Could you check a few things on this model? Use its own coordinates, in mm. A direction names the side the tool comes from. Give positions to 0.01 mm unless a question says otherwise; leave off trailing zeros. Loops run counter-clockwise (first coordinate to the right, second up) from the corner with the lowest first, then second, coordinate; pieces in that order, holes last. Notation, with made-up numbers: M 22.25,12.5 L 42.25,12.5 A17 cw 42.25,32.5 Z; hole C 29.5,73 d8. An arc over 180 degrees is marked long. Return JSON: item names as keys, results as strings. Group by question number.
1. If we mould it in two halves opening along X, with no side actions, what happens to faces 4 (the flat face through (39, 3, 10)), 5 (the flat face through (-76.2, -3, 5)), 6 (the flat face through (-2, 3, 10)), 7 (the flat face through (49, 3, 15))? For each: +X half, -X half, draft (parallel to the pull), parting line (faces both ways), or undercut.
2. If we section it at B-B (x = 0): Write out the boundary of the cut face in (y, z), plus the area to 3 significant figures.
3. For faces 1 (the flat face through (-41, 3, 10)), 2 (the flat face through (65, 3, 10)), 3 (the flat face through (-66, 3, 10)), which set-ups out of +Z, -Z, +X, -X, +Y, -Y let a thin tool reach every point of the face, with its end or its side?
4. If we section it at A-A (y = -153.6): Write out the boundary of the cut face in (x, z), plus the area to 3 significant figures.
5. Please list where these lines run through material, in increasing order: line 1 (Y direction, x = 0, z = 5.25); line 2 (Y direction, x = 1, z = 8.25); line 3 (X direction, y = -125.5, z = 12).
6. If we section it at C-C (y = 48.5): Write out the boundary of the cut face in (x, z).
7. For pin 1 (2.5 mm diameter, centred on y = -22.5, z = 12, fed in from -X); pin 2 (4 mm diameter, centred on y = -43, z = 12.5, fed in from +X); pin 3 (12 mm diameter, centred on x = 0, y = -153.6, fed in from +Z); pin 4 (3 mm diameter, centred on x = -40.5, y = 113.5, fed in from +Z), each with a flat end and sliding along its axis, tell me the tip position at first contact or that it passes through.
```python
from build123d import *

# Parameters (mm, degrees)
SKETCH1_W           = 152.4
SKETCH1_H           = 457.2
SKETCH1_R           = 10
BOSS_EXTRUDE1_DEPTH = 10
SKETCH2_W           = 10
SKETCH2_H           = 457.2
EXTRUDE_THIN1_DEPTH = 5


with BuildPart() as part:
    # Sketch1 → Boss-Extrude1 (new body)
    with BuildSketch(Plane.XY):
        Rectangle(SKETCH1_W, SKETCH1_H)
        with Locations((0, -203.6)):
            Circle(SKETCH1_R, mode=Mode.SUBTRACT)
        with Locations((0, -153.6)):
            Circle(SKETCH1_R, mode=Mode.SUBTRACT)
    extrude(amount=BOSS_EXTRUDE1_DEPTH)

    # Sketch2 → Extrude-Thin1 (add)
    with BuildSketch(Plane.XY.offset(10)):
        with Locations((28.665766577, 0)):
            Rectangle(SKETCH2_W, SKETCH2_H)
        with Locations((48.665766577, 0)):
            Rectangle(SKETCH2_W, SKETCH2_H)
        with Locations((-31.334233423, 0)):
            Rectangle(SKETCH2_W, SKETCH2_H)
        with Locations((-51.334233423, 0)):
            Rectangle(SKETCH2_W, SKETCH2_H)
    extrude(amount=EXTRUDE_THIN1_DEPTH)


solid = part.part
```
Answer:
{
 "1": {"face 4": "undercut", "face 5": "-X half", "face 6": "undercut", "face 7": "draft"},
 "2": {"outline": "M -228.6,0 L -213.6,0 L -213.6,10 L -228.6,10 Z; M -193.6,0 L -163.6,0 L -163.6,10 L -193.6,10 Z; M -143.6,0 L 228.6,0 L 228.6,10 L -143.6,10 Z", "area": "4,170 mm²"},
 "3": {"face 1": "+Z, +Y, -Y", "face 2": "+Z, +X, +Y, -Y", "face 3": "+Z, -X, +Y, -Y"},
 "4": {"outline": "M -76.2,0 L -10,0 L -10,10 L -26.33,10 L -26.33,15 L -36.33,15 L -36.33,10 L -46.33,10 L -46.33,15 L -56.33,15 L -56.33,10 L -76.2,10 Z; M 10,0 L 76.2,0 L 76.2,10 L 53.67,10 L 53.67,15 L 43.67,15 L 43.67,10 L 33.67,10 L 33.67,15 L 23.67,15 L 23.67,10 L 10,10 Z", "area": "1,520 mm²"},
 "5": {"line 1": "y = -228.6 to -213.6, -193.6 to -163.6, -143.6 to 228.6", "line 2": "y = -228.6 to -213.55, -193.65 to -163.55, -143.65 to 228.6", "line 3": "x = -56.33 to -46.33, -36.33 to -26.33, 23.67 to 33.67, 43.67 to 53.67"},
 "6": {"outline": "M -76.2,0 L 76.2,0 L 76.2,10 L 53.67,10 L 53.67,15 L 43.67,15 L 43.67,10 L 33.67,10 L 33.67,15 L 23.67,15 L 23.67,10 L -26.33,10 L -26.33,15 L -36.33,15 L -36.33,10 L -46.33,10 L -46.33,15 L -56.33,15 L -56.33,10 L -76.2,10 Z"},
 "7": {"pin 1": "stops at x = -56.33", "pin 2": "stops at x = 53.67", "pin 3": "passes through", "pin 4": "stops at z = 10"}
}
